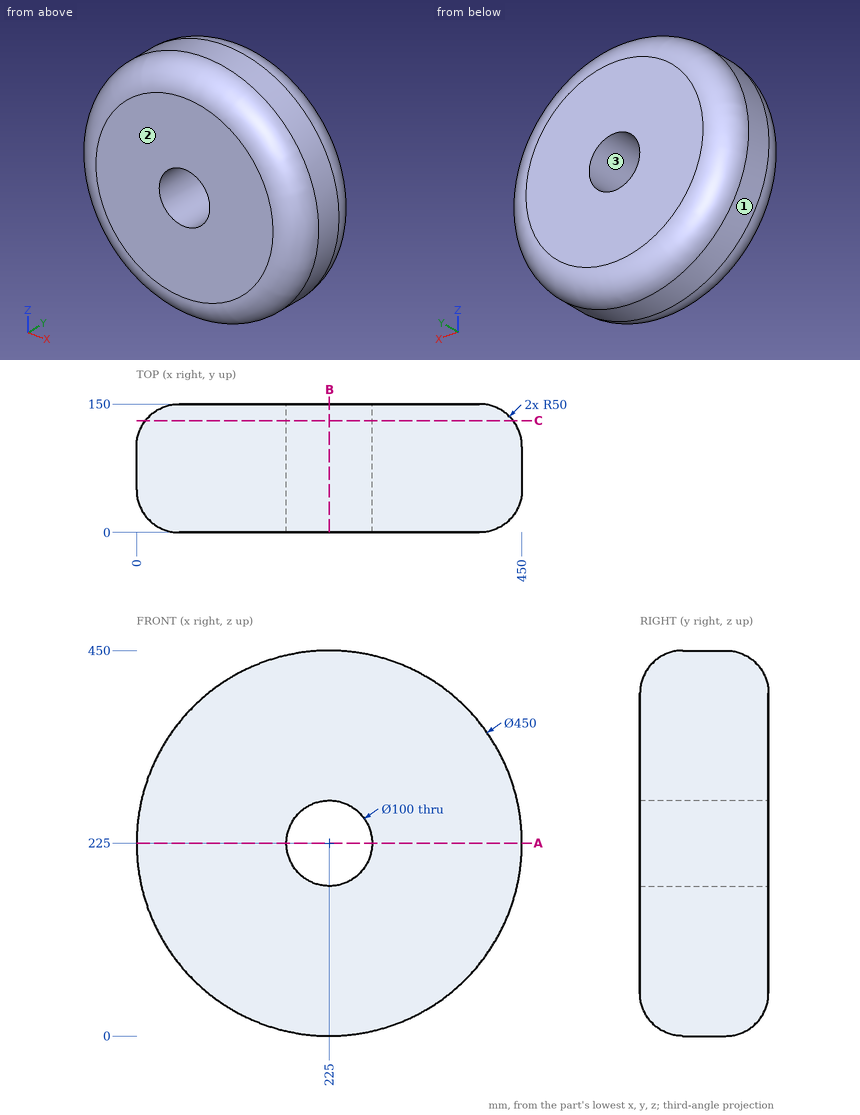
Verification items for this drawing (mm, ordinates from the low corner). Give positions to 0.01 mm unless a question says otherwise; leave off trailing zeros. Loops run counter-clockwise (first coordinate to the right, second up) from the corner with the lowest first, then second, coordinate; pieces in that order, holes last.
(1) Section check B-B on x = 225. Record the cut outline in (y, z).
From the geometry:
outline: (0, 50) arc R50 ccw to (50, 0) - (100, 0) arc R50 ccw to (150, 50) - (150, 175) - (0, 175) - close; (0, 275) - (150, 275) - (150, 400) arc R50 ccw to (100, 450) - (50, 450) arc R50 ccw to (0, 400) - close
(2) Release check for a two-part mould opening along X. For the marked faces 1, 2 and 3 record: released by +X, released by -X, zero draft, split by the parting line, or undercut.
From the geometry:
face 1: split by the parting line
face 2: zero draft
face 3: undercut
(3) Section check C-C on y = 130.5. Record the cut outline in (x, z).
From the geometry:
outline: circle Ø429.24 at (225, 225); hole circle Ø100 at (225, 225)
(4) Thickness scan on L1, parallel to Z at x = 225, y = 100; L2, parallel to X at y = 44, z = 229.5; L3, parallel to X at y = 82, z = 204. Record the ranges inside material, lowest first.
From the geometry:
L1: z = 0 to 175, 275 to 450
L2: x = 0.41 to 175.2, 274.8 to 449.59
L3: x = 0.98 to 179.62, 270.38 to 449.02
(5) Depth check by flat-ended pin: pin 1 Ø3 at (x, y) = (349, 133) entering from +Z; pin 2 Ø4 at (y, z) = (90, 141) entering from -X; pin 3 Ø5 at (y, z) = (117.5, 363.5) entering from +X; pin 4 Ø10 at (x, z) = (179.5, 375.5) entering from -Y. Enter the tip coordinate at first touch or a pass-through.
From the geometry:
pin 1: stops at z = 399.54
pin 2: stops at x = 15.47
pin 3: stops at x = 400.57
pin 4: stops at y = 0
(6) Section check A-A on z = 225. Record the cut outline in (x, y).
From the geometry:
outline: (0, 50) arc R50 ccw to (50, 0) - (175, 0) - (175, 150) - (50, 150) arc R50 ccw to (0, 100) - close; (275, 0) - (400, 0) arc R50 ccw to (450, 50) - (450, 100) arc R50 ccw to (400, 150) - (275, 150) - close
